Source: three-view drawing plus pictorial views. Frame: mm from the lowest corner of the part. Give positions to 0.01 mm unless a question says otherwise; leave off trailing zeros. Loops run counter-clockwise (first coordinate to the right, second up) from the corner with the lowest first, then second, coordinate; pieces in that order, holes last. Notation, with made-up numbers: M 45,87 L 60,87 A28 cw 60,119 Z; hole C 40.5,-38 d11. An arc over 180 degrees is marked long. Answer as a JSON object with one key per item and string values. Group by question number.
1) Ray query, L1, parallel to X at y = 201.5, z = 187; L2, parallel to Y at x = 307, z = 302.5. Return the intervals inside material, ascending.
2) Section query B-B on z = 343.5. Return loops of the section in (x, y).
3) Section query A-A on x = 493. Return loops of the section in (y, z), plus the area to 3 significant figures.
4) First-contact query: P1, Ø12.5, axis at x = 13.5, z = 65.5, coming from the -Y side; P2, Ø7.5, axis at x = 621, y = 199.5, coming from the -Z side. Flat tips, straight axial feed; report the tip coordinate or a pass-through.
5) Section query C-C on z = 136.5. Return loops of the section in (x, y), plus the area to 3 significant figures.
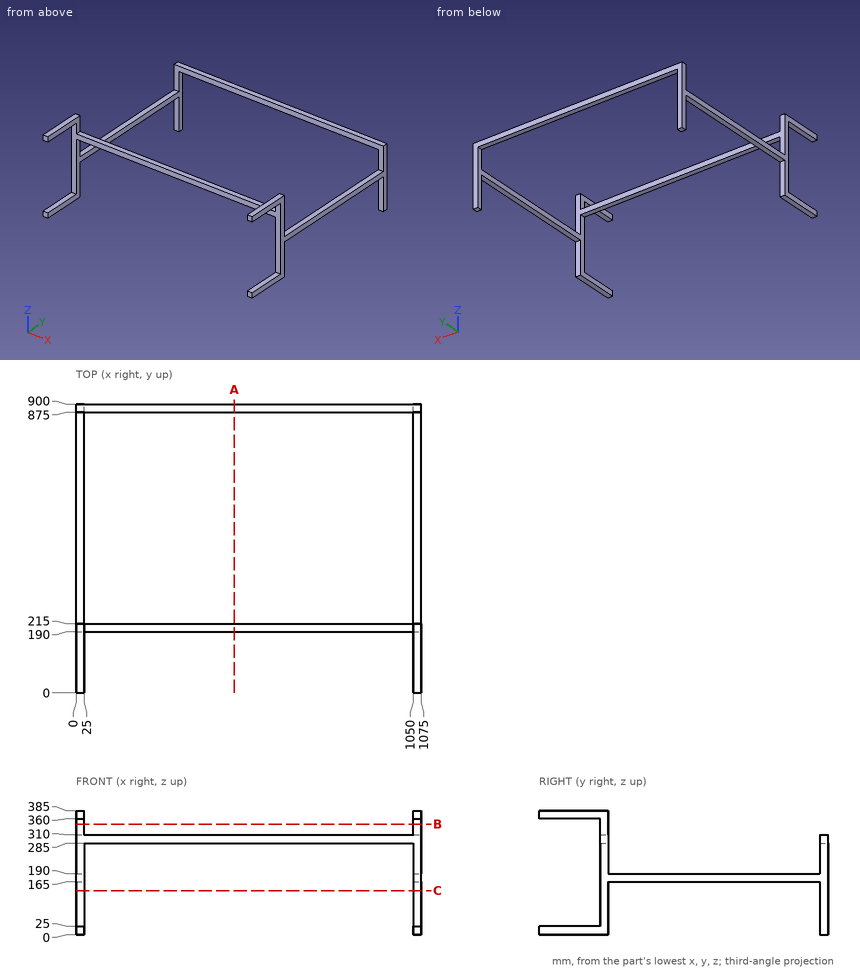
Output:
{
 "1": {"L1": "x = 0 to 25, 1050 to 1075", "L2": "y = 190 to 215, 875 to 900"},
 "2": {"outline": "M 0,190 L 25,190 L 25,215 L 0,215 Z; M 1050,190 L 1075,190 L 1075,215 L 1050,215 Z"},
 "3": {"outline": "M 190,285 L 215,285 L 215,310 L 190,310 Z; M 875,285 L 900,285 L 900,310 L 875,310 Z", "area": "1,250 mm^2"},
 "4": {"P1": "stops at y = 190", "P2": "stops at z = 285"},
 "5": {"outline": "M 0,190 L 25,190 L 25,215 L 0,215 Z; M 0,875 L 25,875 L 25,900 L 0,900 Z; M 1050,190 L 1075,190 L 1075,215 L 1050,215 Z; M 1050,875 L 1075,875 L 1075,900 L 1050,900 Z", "area": "2,500 mm^2"}
}
